Read the model definition and answer for the solid it produces. Units are mm, in the model's axes. A direction names the side the tool comes from. Coordinates: 2 decimals unless noted, no trailing zeros. Loops run counter-clockwise (first coordinate to the right, second up) from the corner with the lowest first, then second, coordinate; pieces in that order, holes last.
Q1. Section A-A (z = -4.5) is taken. Give the vertices of the cut face in (x, y).
Q2. The mould has two halves that part along Y. Classify faces 3 (the face through (-4, 50.8, 0)), 4 (the face through (-84.54, 3.96, -3.93)), 5 (the face through (4.27, -42.97, -0.11)), 6 (the face through (-304.8, -1, 0)): pulls with the +Y half, pulls with the -Y half, needs draft (parallel to the pull), parting line crosses it, or undercut.
Q3. Straight lines are drawn through the part: line 1 (X direction, y = -3, z = 3.25); line 2 (X direction, y = 4, z = 5.5); line 3 (Y direction, x = 234.95, z = 2.75). For each, find the intervals that lie inside material, in ascending order.
Q4. Section B-B (x = -210.5) is taken. Give the vertices of the cut face in (y, z) (1 decimal).
Q5. Flat-ended cylindrical pins translate along their axes: P1, Ø11, axis at x = 71.97, y = 0, coming from the +Z side; P2, Ø8.5, axis at x = 234.95, y = 0, coming from the -Z side; P3, Ø23.5, axis at x = -71.97, y = 0, coming from the -Z side. Find the tip coordinate at first contact, or state that the pin passes through.
Q6. Which of the six approach directions +Z, -Z, +X, -X, +Y, -Y give full straight-line access (tool end or side, diameter ignored) to faces 1 (the face through (222.773, -5.049, -3.93)), 2 (the face through (-4, 1, -7.938))?
from build123d import *

# Parameters (mm, degrees)
SKETCH1_W               = 609.6
SKETCH1_H               = 101.6
BOSS_EXTRUDE1_DEPTH     = 7.9375
CUT_EXTRUDE2_DEPTH      = 1
CUT_EXTRUDE2_DEPTH_BACK = 610.6
SKETCH4_R               = 4.826
CUT_EXTRUDE3_DEPTH      = 1
CUT_EXTRUDE3_DEPTH_BACK = 16.875
SKETCH4_3_R             = 13.1826
SKETCH4_3_R_2           = 4.826
CUT_EXTRUDE4_DEPTH      = 8.128


with BuildPart() as part:
    # Sketch1 → Boss-Extrude1 (new body, symmetric)
    with BuildSketch(Plane.XY):
        Rectangle(SKETCH1_W, SKETCH1_H)
    extrude(amount=BOSS_EXTRUDE1_DEPTH, both=True)

    # Sketch3 → Cut-Extrude2 (cut, two sides)
    with BuildSketch(Plane(origin=(304.8, 0, 0), x_dir=(0, 0, -1), z_dir=(1, 0, 0))) as cut_extrude2_sk:
        Polygon((7.9375, -50.8), (-7.9375, -34.925), (-7.9375, -50.8), align=None)
    extrude(amount=CUT_EXTRUDE2_DEPTH, mode=Mode.SUBTRACT)
    extrude(cut_extrude2_sk.sketch, amount=-CUT_EXTRUDE2_DEPTH_BACK, mode=Mode.SUBTRACT)

    # Sketch4 → Cut-Extrude3 (cut, two sides)
    with BuildSketch(Plane(origin=(0, 0, -7.9375), x_dir=(-1, 0, 0), z_dir=(0, 0, -1))) as cut_extrude3_sk:
        with Locations((-234.95, 0)):
            Circle(SKETCH4_R)
        with Locations((-71.966666709, 0)):
            Circle(SKETCH4_R)
        with Locations((71.966666709, 0)):
            Circle(SKETCH4_R)
        with Locations((234.95, 0)):
            Circle(SKETCH4_R)
    extrude(amount=CUT_EXTRUDE3_DEPTH, mode=Mode.SUBTRACT)
    extrude(cut_extrude3_sk.sketch, amount=-CUT_EXTRUDE3_DEPTH_BACK, mode=Mode.SUBTRACT)

    # Sketch4<3> → Cut-Extrude4 (cut)
    with BuildSketch(Plane(origin=(0, 0, -7.9375), x_dir=(-1, 0, 0), z_dir=(0, 0, -1))):
        with Locations((-234.95, 0)):
            Circle(SKETCH4_3_R)
        with Locations((-234.95, 0)):
            Circle(SKETCH4_3_R_2, mode=Mode.SUBTRACT)
        with Locations((-71.966666709, 0)):
            Circle(SKETCH4_3_R)
        with Locations((-71.966666709, 0)):
            Circle(SKETCH4_3_R_2, mode=Mode.SUBTRACT)
        with Locations((234.95, 0)):
            Circle(SKETCH4_3_R)
        with Locations((234.95, 0)):
            Circle(SKETCH4_3_R_2, mode=Mode.SUBTRACT)
        with Locations((71.966666709, 0)):
            Circle(SKETCH4_3_R)
        with Locations((71.966666709, 0)):
            Circle(SKETCH4_3_R_2, mode=Mode.SUBTRACT)
    extrude(amount=-CUT_EXTRUDE4_DEPTH, mode=Mode.SUBTRACT)


solid = part.part
Numbers:
1. outline: (-304.8, -47.36) - (304.8, -47.36) - (304.8, 50.8) - (-304.8, 50.8) - close; hole circle Ø26.37 at (-234.95, 0); hole circle Ø26.37 at (-71.97, 0); hole circle Ø26.37 at (71.97, 0); hole circle Ø26.37 at (234.95, 0)
2. face 3: pulls with the +Y half
2. face 4: undercut
2. face 5: pulls with the -Y half
2. face 6: needs draft
3. line 1: x = -304.8 to -238.73, -231.17 to -75.75, -68.19 to 68.19, 75.75 to 231.17, 238.73 to 304.8
3. line 2: x = -304.8 to -237.65, -232.25 to -74.67, -69.27 to 69.27, 74.67 to 232.25, 237.65 to 304.8
3. line 3: y = -40.11 to -4.83, 4.83 to 50.8
4. outline: (-50.8, -7.9) - (50.8, -7.9) - (50.8, 7.9) - (-34.9, 7.9) - close
5. P1: stops at z = 7.94
5. P2: passes through
5. P3: stops at z = 0.19
6. face 1: -Z
6. face 2: -Z, +X, -X, +Y, -Y
